Can you work these out from the model? Positions are in its coordinate system, mm. Face numbers are marked on the shaded views. A direction names the side the tool comes from. Round coordinates to 2 decimals unless told otherwise and drop trailing zeros. Loops run counter-clockwise (first coordinate to the right, second up) from the corner with the lowest first, then second, coordinate; pieces in that order, holes last. Notation, with made-up numbers: (18, 62) -> (69, 62) arc R18 cw to (69, 75) -> close; hole circle Ø5 at (9.25, 35.25). An arc over 180 degrees is marked (long way). Answer as a JSON object with one key per item and string values.
```python
from build123d import *

# Parameters (mm, degrees)
F1_DEPTH  = 16
F2_W      = 70
F2_H      = 3
F3_DEPTH  = 2
F4_W      = 50
F4_H      = 14
F5_DEPTH  = 2
F6_R      = 1
F9_DEPTH  = 2
F11_DEPTH = 42.001
F13_D     = 4
F14_R     = 3
F14_R_2   = 2
F15_DEPTH = 5
F17_R     = 5


with BuildPart() as f1:
    # F0 (on Front) → F1 (new body)
    with BuildSketch(Plane.XZ):
        with BuildLine():
            Line((94, 11), (0, 11))
            ThreePointArc((0, 11), (-11, 0), (0, -11))
            Line((0, -11), (19, -11))
            ThreePointArc((19, -11), (21.7681124643, -11.8361612201), (23.6103896104, -14.064978646))
            ThreePointArc((23.6103896104, -14.064978646), (52.4237101957, -47.6174640031), (95.4149528414, -57.9967593826))
            ThreePointArc((95.4149528414, -57.9967593826), (101.3804745105, -59.0597282402), (106.3380534538, -62.5439444501))
            Line((106.3380534538, -62.5439444501), (107.6335766724, -61))
            ThreePointArc((107.6335766724, -61), (102.0097459375, -57.1560789275), (95.2965735981, -56))
            ThreePointArc((95.2965735981, -56), (53.4811996085, -45.9198240056), (25.4545454545, -13.2909701044))
            ThreePointArc((25.4545454545, -13.2909701044), (22.87535745, -10.1706257081), (19, -9))
            Line((19, -9), (0, -9))
            ThreePointArc((0, -9), (-9, 0), (0, 9))
            Line((0, 9), (94, 9))
            Line((94, 9), (94, 11))
        make_face()
    extrude(amount=F1_DEPTH)

    # F2 (on face) → F3 (join)
    with BuildSketch(Plane.XY.offset(11)):
        with Locations((59, -17.5)):
            Rectangle(F2_W, F2_H)
    extrude(amount=-F3_DEPTH)

    # F4 (on face) → F5 (join)
    with BuildSketch(Plane.XZ.offset(19)):
        with Locations((69, 4)):
            Rectangle(F4_W, F4_H)
    extrude(amount=F5_DEPTH)

    # F6
    f6_edges = [f1.edges().sort_by_distance(p)[0] for p in [
        (69, -21, 11),
        (69, -19, 9),
    ]]
    fillet(f6_edges, radius=F6_R)

    # F7: F1 across plane


with BuildPart() as f1_1:
    add(f1.part)
    add(f1.part.mirror(Plane.XZ))

    # F8 (on face) → F9 (cut)
    with BuildSketch(Plane.XY.offset(11)):
        with BuildLine():
            Line((94, 12), (34, 12))
            ThreePointArc((34, 12), (22, 0), (34, -12))
            Line((34, -12), (94, -12))
            Line((94, -12), (94, 12))
        make_face()
    extrude(amount=-F9_DEPTH, mode=Mode.SUBTRACT)

    # F10 (on face) → F11 (cut, through all)
    with BuildSketch(Plane(origin=(0, 21, 0), x_dir=(-1, 0, 0), z_dir=(0, 1, 0))):
        with BuildLine():
            ThreePointArc((-70, 8), (-73, 5), (-70, 2))
            Line((-70, 2), (-50, 2))
            ThreePointArc((-50, 2), (-47, 5), (-50, 8))
            Line((-50, 8), (-70, 8))
        make_face()
    extrude(amount=-F11_DEPTH, mode=Mode.SUBTRACT)

    # F13 (through all)
    with Locations(Plane(origin=(0, 21, 0), x_dir=(-1, 0, 0), z_dir=(0, 1, 0))):
        with Locations((-80, 3)):
            Hole(F13_D / 2)

    # F14 (on face) → F15 (join)
    with BuildSketch(Plane.XZ.offset(-19)):
        with Locations((80, 3)):
            Circle(F14_R)
        with Locations((80, 3)):
            Circle(F14_R_2, mode=Mode.SUBTRACT)
    extrude(amount=F15_DEPTH)

    # F16: F1 across plane


with BuildPart() as f1_2:
    add(f1_1.part)
    add(f1_1.part.mirror(Plane.XZ))

    # F17
    f17_edges = [f1_2.edges().sort_by_distance(p)[0] for p in [
        (94, 20, -3),
        (44, 20, -3),
        (94, -20, -3),
        (44, -20, -3),
    ]]
    fillet(f17_edges, radius=F17_R)


solid = f1_2.part
```
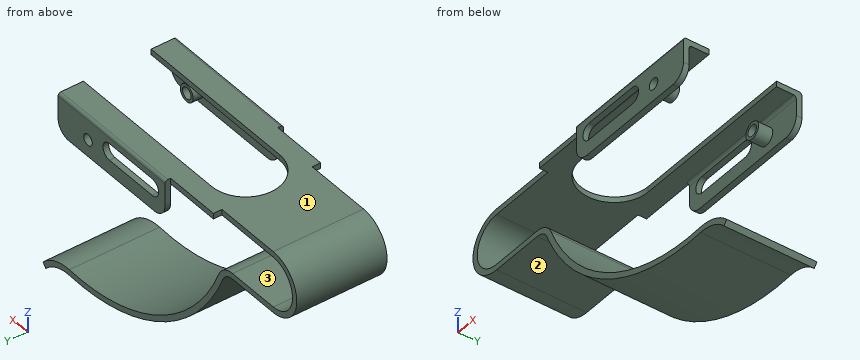
Q1. I want a section at B-B, the plane y = -3. Write out the boundary of the cut face in (x, z), then the cut area to 3 significant figures.
Determined:
{"outline": "(0, -11) -> (19, -11) arc R5 cw to (23.61, -14.06) arc R72 ccw to (95.41, -58) arc R14 cw to (106.34, -62.54) -> (107.63, -61) arc R16 ccw to (95.3, -56) arc R70 cw to (25.45, -13.29) arc R7 ccw to (19, -9) -> (0, -9) arc R9 cw to (0, 9) -> (22.38, 9) -> (22.38, 11) -> (0, 11) arc R11 ccw to start", "area": "363 mm²"}
Q2. I want a section at D-D, the plane z = -33. Write out the boundary of the cut face in (x, y), then the cut area to 3 significant figures.
Determined:
{"outline": "(35.28, -16) -> (37.94, -16) -> (37.94, 16) -> (35.28, 16) -> close", "area": "85.1 mm²"}
Q3. If I drill on L1, parallel to Z at x = 80, y = 20.1; L2, parallel to Z at x = 12, y = 10.5; L3, parallel to X at y = 6.5, z = 0.5, over which ranges is the centre line in solid material (lowest first)? Write a range as [from, to].
Determined:
{"L1": "[-3, 1], [5, 10.99]", "L2": "[-11, -9], [9, 11]", "L3": "[-10.99, -8.99]"}
Q4. On a 3-axis mill with a long thin cutter (end or side, diameter ignored), from which of +Z, -Z, +X, -X, +Y, -Y can I reach the whole of each face in a straight line? I mean the marked faces 1, 2 and 3. Say none if no direction works.
Determined:
{"face 1": "+Z, +X, -X, +Y, -Y", "face 2": "-Z, -X, +Y, -Y", "face 3": "+X, +Y, -Y"}
Q5. I want a section at A-A, the plane x = 54. Write out the boundary of the cut face in (y, z), then the cut area to 3 significant figures.
Determined:
{"outline": "(-21, -3) -> (-19, -3) -> (-19, 2) -> (-21, 2) -> close; (-21, 8) -> (-19, 8) arc R1 cw to (-18, 9) -> (-12, 9) -> (-12, 11) -> (-20, 11) arc R1 ccw to (-21, 10) -> close; (-16, -48.55) -> (16, -48.55) -> (16, -46.23) -> (-16, -46.23) -> close; (12, 9) -> (18, 9) arc R1 cw to (19, 8) -> (21, 8) -> (21, 10) arc R1 ccw to (20, 11) -> (12, 11) -> close; (19, -3) -> (21, -3) -> (21, 2) -> (19, 2) -> close", "area": "134 mm²"}
Q6. I want a section at C-C, the plane x = -2.5. Write out the boundary of the cut face in (y, z).
Determined:
{"outline": "(-16, -10.71) -> (16, -10.71) -> (16, -8.65) -> (-16, -8.65) -> close; (-16, 8.65) -> (16, 8.65) -> (16, 10.71) -> (-16, 10.71) -> close"}
Q7. I'm going to push flat-ended pins straight in: pin 1 (0.6 mm diameter, centred on x = 59.5, y = -20.5, fed in from -Z); pin 2 (2 mm diameter, centred on y = -4.5, z = -45, fed in from -X); pin 3 (5.5 mm diameter, centred on x = 10.5, y = -2.5, fed in from -Z). Where does each tip first touch, or does it pass through?
Determined:
{"pin 1": "z = -3", "pin 2": "x = 47.07", "pin 3": "z = -11"}
